Build history of the part. All positions in model axes, mm. A direction names the side the tool comes from. Round coordinates to 2 decimals unless told otherwise and drop trailing zeros. Loops run counter-clockwise (first coordinate to the right, second up) from the corner with the lowest first, then second, coordinate; pieces in that order, holes last. Notation, with made-up numbers: (-33.5, 64.5) -> (-7.5, 64.5) arc R38 cw to (-7.5, 103.5) -> close; hole circle Ø2 at (64.25, -1.5). An arc over 180 degrees is marked (long way). Put each result on its own line as item: value. Start each with the question number.
```python
from build123d import *

# Parameters (mm, degrees)
SKETCH2_R          = 1.75
CUT_EXTRUDE1_DEPTH = 14
FILLET1_R          = 0.5


with BuildPart() as part:
    # Sketch1 → Revolve1 (revolve)
    with BuildSketch(Plane.XY):
        Polygon((-6.5, 0), (-6.5, 4.25), (-5, 4.25), (-5, 3), (-3.25, 3), (-3.25, 4.25), (3.25, 4.25), (3.25, 3), (5, 3), (5, 4.25), (6.5, 4.25), (6.5, 0), align=None)
    revolve(axis=Axis((6.5, 0, 0), (-1, 0, 0)))

    # Sketch2 → Cut-Extrude1 (cut, through all)
    with BuildSketch(Plane(origin=(6.5, 0, 0), x_dir=(0, 0, -1), z_dir=(1, 0, 0))):
        Circle(SKETCH2_R)
    extrude(amount=-CUT_EXTRUDE1_DEPTH, mode=Mode.SUBTRACT)

    # Fillet1
    fillet1_edges = [part.edges().sort_by_distance(p)[0] for p in [
        (3.25, -4.25, 0),
        (-3.25, -4.25, 0),
    ]]
    fillet(fillet1_edges, radius=FILLET1_R)


solid = part.part
```
Item 1: 3-axis set-ups, long thin cutter, end or side, ignore diameter. For faces 1 (the face through (0.091, -0.67, -1.617)), 2 (the face through (5, -1, -3)): which of +Z, -Z, +X, -X, +Y, -Y reach the whole face in a straight line?
Item 2: Cut at C-C on x = 5.5. Write the cut outline in (y, z), then the cut area to 3 significant figures.
Item 3: Cut at D-D on x = -4.25. Write the cut outline in (y, z), then the cut area to 3 significant figures.
Item 4: Pull direction X, two halves, no side cores. Call faces 3 (the face through (-6.5, -2, 0)), 4 (the face through (-3.25, -1, -3)), 5 (the face through (6.5, 2, 0)): +X half, -X half, draft (parallel to the pull), parting line (faces both ways), or undercut.
Item 5: Drop flat-ended pins along their axis: pin 1 (3 mm diameter, centred on y = 1.5, z = 0, fed in from +X); pin 2 (3 mm diameter, centred on x = 1.5, y = 3, fed in from +Z). Give the stop position or say it passes through.
Item 6: Cut at A-A on z = 0. Write the cut outline in (x, y), then the cut area to 3 significant figures.
Item 7: Wall check: line 1 (X direction, y = 0.25, z = -3.5); line 2 (Y direction, x = 3.75, z = 0); line 3 (Y direction, x = -1.5, z = 0). Give the ranges that are in metal, low to high. Write a range as from..to.
Ans:
1. face 1: +X, -X
1. face 2: none
2. outline: circle Ø8.5 at (0, 0); hole circle Ø3.5 at (0, 0)
2. area: 47.1 mm2
3. outline: circle Ø6 at (0, 0); hole circle Ø3.5 at (0, 0)
3. area: 18.7 mm2
4. face 3: -X half
4. face 4: undercut
4. face 5: +X half
5. pin 1: stops at x = 6.5
5. pin 2: stops at z = 3.98
6. outline: (-6.5, -4.25) -> (-5, -4.25) -> (-5, -3) -> (-3.25, -3) -> (-3.25, -3.75) arc R0.5 ccw to (-2.75, -4.25) -> (2.75, -4.25) arc R0.5 ccw to (3.25, -3.75) -> (3.25, -3) -> (5, -3) -> (5, -4.25) -> (6.5, -4.25) -> (6.5, -1.75) -> (-6.5, -1.75) -> close; (-6.5, 1.75) -> (6.5, 1.75) -> (6.5, 4.25) -> (5, 4.25) -> (5, 3) -> (3.25, 3) -> (3.25, 3.75) arc R0.5 ccw to (2.75, 4.25) -> (-2.75, 4.25) arc R0.5 ccw to (-3.25, 3.75) -> (-3.25, 3) -> (-5, 3) -> (-5, 4.25) -> (-6.5, 4.25) -> close
6. area: 56.0 mm2
7. line 1: x = -6.5..-5, -3.25..3.25, 5..6.5
7. line 2: y = -3..-1.75, 1.75..3
7. line 3: y = -4.25..-1.75, 1.75..4.25
